For this review, take the finished solid that the model builds, in its own axes (mm). Face numbers are marked on the shaded views. A direction names the side the tool comes from. Give positions to 0.01 mm unless a question says otherwise; leave off trailing zeros. Loops run counter-clockwise (first coordinate to the right, second up) from the corner with the lowest first, then second, coordinate; pieces in that order, holes last. Notation, with made-up numbers: M 9,28 L 61,28 A5 cw 61,36 Z; hole C -25.5,-12 d7. An arc over 180 degrees is marked long. Use CSV: the item, a comma, the result in double quotes. Start each with the question number.
1. Tool access review of the marked faces 5 and 6: name each direction out of +Z, -Z, +X, -X, +Y, -Y from which nothing blocks a thin tool from reaching the whole face with its end or side.
2. The part is to be moulded in two halves that separate along Z. For the marked faces 1, 2, 3 and 4, say which applies: pulls with the +Z half, pulls with the -Z half, needs draft (parallel to the pull), parting line crosses it, or undercut.
3. Insertion check: P1, Ø1, axis at x = 6, z = 57.5, coming from the -Y side; P2, Ø14.5, axis at x = -3, y = 38.5, coming from the -Z side; P3, Ø6.5, axis at x = 11.5, y = 30, coming from the +Z side; P4, Ø2, axis at x = 12, y = 7, coming from the -Z side. Each pin has a flat end and moves straight along its axis. Give the tip position at first contact, or say it passes through.
4. Take a section at B-B, the plane z = -9. Write out the cut boundary in (x, y) (3 decimals), and give its area (3 significant figures).
5. Take a section at A-A, the plane y = 32.5. Write out the cut boundary in (x, z).
6. To check wall thickness, follow line 1 (Z direction, x = 7, y = 33.5); line 2 (Y direction, x = -10, z = 2.5); line 3 (Z direction, x = 4.5, y = 15). State the ranges of each line that lie inside material, in increasing order. Write a range as [from, to].
7. Take a section at C-C, the plane x = -10. State how many separate pieces and enclosed holes the cut face has, and give its area (3 significant figures).
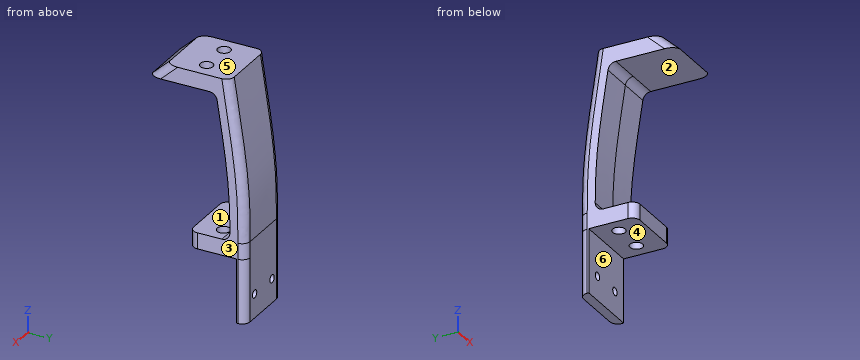
from build123d import *

# Parameters (mm, degrees)
SKETCH1_W           = 40
SKETCH1_H           = 120
BOSS_EXTRUDE1_DEPTH = 10
LOFT1_START         = -20
LOFT1_DEPTH         = 40
CUT_EXTRUDE2_DEPTH  = 109
FILLET2_R           = 5
SKETCH7_R           = 4
CUT_EXTRUDE3_DEPTH  = 5
SKETCH8_R           = 4
CUT_EXTRUDE4_DEPTH  = 10
FILLET4_R           = 5
BOSS_EXTRUDE3_DEPTH = 40
SKETCH10_R          = 2.5
CUT_EXTRUDE5_DEPTH  = 10


# Read off the part's stored shape, not the designer's step: Loft1
with BuildPart() as part:
    # Sketch1 → Boss-Extrude1 (new body)
    with BuildSketch(Plane.XY):
        Rectangle(SKETCH1_W, SKETCH1_H)
    extrude(amount=BOSS_EXTRUDE1_DEPTH)

    # Loft1 outline → Loft1 (add)
    with BuildSketch(Plane.YZ.offset(LOFT1_START)):
        with BuildLine():
            add(Edge.make_bspline(
                [(-60, 10), (-60, 30.441311123), (-60, 50.882622246), (-32, 70.441311123), (-11, 90.220655562), (10, 110)],
                knots=[0, 0, 0, 0, 0, 0, 1, 1, 1, 1, 1, 1], degree=5))
            Line((-60, 10), (60, 10))
            add(Edge.make_bspline(
                [(60, 10), (60, 30.009975124), (60, 50.019950248), (56, 70.009975124), (53, 90.004987562), (50, 110)],
                knots=[0, 0, 0, 0, 0, 0, 1, 1, 1, 1, 1, 1], degree=5))
            Line((50, 110), (10, 110))
        make_face()
    extrude(amount=LOFT1_DEPTH)

    # Sketch5 → Cut-Extrude2 (cut, symmetric)
    with BuildSketch(Plane(origin=(0, 0, 0), x_dir=(0, 0, -1), z_dir=(1, 0, 0))):
        with BuildLine():
            Line((0, -60), (-100, -60))
            Line((-100, -60), (-100, 41.393396846))
            add(Edge.make_bspline(
                [(-10, 50), (-14.168744818, 50), (-18.275601874, 49.996409138), (-26.428009759, 49.87077255), (-30.473567498, 49.749630948), (-38.552130932, 49.347381325), (-42.585186542, 49.066850503), (-50.67278015, 48.349847693), (-54.727313877, 47.913843652), (-62.876208691, 46.920588729), (-66.970526782, 46.363844017), (-75.202509115, 45.180338869), (-79.340154976, 44.554169827), (-87.648626866, 43.2832223), (-91.819473021, 42.639096286), (-97.329708937, 41.798417087), (-98.664929704, 41.595568065), (-100, 41.393396846)],
                knots=[0, 0, 0, 0, 0.125, 0.125, 0.25, 0.25, 0.375, 0.375, 0.5, 0.5, 0.625, 0.625, 0.75, 0.75, 0.875, 0.875, 0.914957714, 0.914957714, 0.914957714, 0.914957714], degree=3))
            Line((-10, 50), (-10, 24.6))
            Line((-10, 24.6), (0, 24.6))
            Line((0, 24.6), (0, -60))
        make_face()
    extrude(amount=CUT_EXTRUDE2_DEPTH, both=True, mode=Mode.SUBTRACT)

    # Fillet2
    fillet2_edges = [part.edges().sort_by_distance(p)[0] for p in [
        (20, 60, 5),
        (-20, 60, 5),
        (20, 4.6735266, 104.990679985),
        (-20, 4.6735266, 104.990679985),
        (-20, 57.319131326, 60.213292337),
        (20, 57.319131326, 60.213292337),
    ]]
    fillet(fillet2_edges, radius=FILLET2_R)

    # Sketch7 → Cut-Extrude3 (cut)
    with BuildSketch(Plane.XY.offset(110)):
        with Locations((-10, 30)):
            Circle(SKETCH7_R)
        with Locations(Location((10, 30, 0), (0, 0, 270))):
            Circle(SKETCH7_R)
        with Locations((10, -30)):
            Circle(SKETCH7_R)
        with Locations((-10, -30)):
            Circle(SKETCH7_R)
    extrude(amount=-CUT_EXTRUDE3_DEPTH, mode=Mode.SUBTRACT)

    # Sketch8 → Cut-Extrude4 (cut)
    with BuildSketch(Plane(origin=(0, 0, 0), x_dir=(-1, 0, 0), z_dir=(0, 0, -1))):
        with Locations((-10, 40.6)):
            Circle(SKETCH8_R)
        with Locations(Location((10, 40.6, 0), (0, 0, 180))):
            Circle(SKETCH8_R)
    extrude(amount=-CUT_EXTRUDE4_DEPTH, mode=Mode.SUBTRACT)

    # Fillet4
    fillet4_edges = [part.edges().sort_by_distance(p)[0] for p in [
        (-20, 24.6, 5),
        (20, 24.6, 5),
        (-10, 50, 10),
        (-10, 41.393396846, 100),
    ]]
    fillet(fillet4_edges, radius=FILLET4_R)

    # Sketch9 → Boss-Extrude3 (add)
    with BuildSketch(Plane(origin=(0, 0, 0), x_dir=(-1, 0, 0), z_dir=(0, 0, -1))):
        with BuildLine():
            Line((-20, 55), (-20, 54.045))
            Line((-20, 54.045), (20, 54.045))
            Line((20, 54.045), (20, 55))
            ThreePointArc((20, 55), (18.535533906, 58.535533906), (15, 60))
            Line((15, 60), (-15, 60))
            ThreePointArc((-15, 60), (-18.535533906, 58.535533906), (-20, 55))
        make_face()
    extrude(amount=BOSS_EXTRUDE3_DEPTH)

    # Sketch10 → Cut-Extrude5 (cut)
    with BuildSketch(Plane(origin=(0, 60, 0), x_dir=(1, 0, 0), z_dir=(0, 1, 0))):
        with Locations(Location((-10, 25, 0), (0, 0, 270))):
            Circle(SKETCH10_R)
        with Locations(Location((10, 25, 0), (0, 0, 270))):
            Circle(SKETCH10_R)
    extrude(amount=-CUT_EXTRUDE5_DEPTH, mode=Mode.SUBTRACT)


solid = part.part
Result set:
1,face 5,"+Z, +X, -X, +Y, -Y"
1,face 6,"-Z, +X, -X, -Y"
2,face 1,"undercut"
2,face 2,"undercut"
2,face 3,"needs draft"
2,face 4,"pulls with the -Z half"
3,P1,"y = 47.51"
3,P2,"z = 0"
3,P3,"z = 110"
3,P4,"z = 100"
4,outline,"M -20,54.045 L 20,54.045 L 20,55 A5 ccw 15,60 L -15,60 A5 ccw -20,55 Z"
4,area,"227 mm2"
5,outline,"M -20,0 L 20,0 L 20,10 L -20,10 Z; M -20,100 L 20,100 L 20,110 L 13.12,110 L 13.12,105 L 6.88,105 L 6.88,110 L -6.88,110 L -6.88,105 L -13.12,105 L -13.12,110 L -20,110 Z"
6,line 1,"[0, 10], [100, 110]"
6,line 2,"[24.6, 36.6], [44.6, 60]"
6,line 3,"[100, 110]"
7,separate pieces,"3"
7,enclosed holes,"0"
7,area,"1,820 mm2"
